Geometry check sheet. Reference: the model listing, model coordinates, mm. Round coordinates to 2 decimals unless told otherwise and drop trailing zeros. Order: outer loops, then holes, each group sorted by start corner. A loop starts at its lowest first (then second) coordinate and runs counter-clockwise, first axis right, second up. Notation, with made-up numbers: (10.5, 20) -> (35.5, 20) arc R30 ccw to (35.5, 54) -> close; hole circle Ø5 at (76.5, 41). An arc over 180 degrees is marked (long way). Use a Markdown table: item, result. Add a question column.
Item 1: Sectioned sample at D-D, the plane x = 47. Record the cut outline in (y, z).
Item 2: Gauge pin test, flat ends, axial feed: pin 1 Ø0.5 at (x, z) = (19, 1) entering from +Y; pin 2 Ø1.5 at (x, z) = (33, 1) entering from -Y. Record the tip position at first contact, or that the pin passes through.
Item 3: Sectioned sample at A-A, the plane x = -30. Record the cut outline in (y, z), and give its area (3 significant figures).
Item 4: Material ranges on probe 1 along X at (y, z) = (4.5, 1.9); probe 2 along X at (y, z) = (-2.5, 2.4); probe 3 along Y at (x, z) = (-30, 1.95), recorded low to high. Write a range as [from, to].
Item 5: Sectioned sample at C-C, the plane x = -11. Record the cut outline in (y, z), and give its area (3 significant figures).
Item 6: Sectioned sample at B-B, the plane z = 1.15. State how many separate pieces and enclosed holes the cut face has, and give its area (3 significant figures).
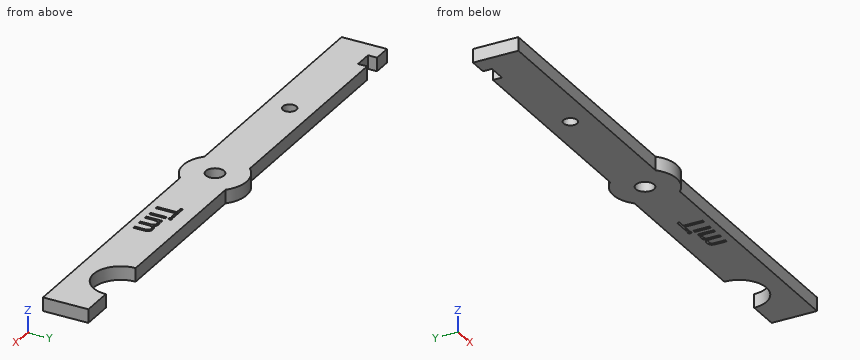
from build123d import *

# Parameters (mm, degrees)
F0_R     = 1.5
F0_R_2   = 2
F0_W     = 0.5472596904
F0_H     = 3.6114921765
F1_DEPTH = 3


with BuildPart() as f1:
    # F0 (on Top) → F1 (new body)
    with BuildSketch(Plane.XY):
        with BuildLine():
            Line((4.8989794856, -5), (-4.8989794856, -5))
            ThreePointArc((-4.8989794856, -5), (0, -7), (4.8989794856, -5))
        make_face()
        with BuildLine():
            ThreePointArc((4.8989794856, 5), (0, 7), (-4.8989794856, 5))
            Line((-4.8989794856, 5), (4.8989794856, 5))
        make_face()
        with BuildLine():
            Line((-60, 5), (-60, -5))
            Line((-60, -5), (-4.8989794856, -5))
            ThreePointArc((-4.8989794856, -5), (-7, 0), (-4.8989794856, 5))
            Line((-4.8989794856, 5), (-52, 5))
            Line((-52, 5), (-52, 3))
            Line((-52, 3), (-56, 3))
            Line((-56, 3), (-56, 5))
            Line((-56, 5), (-60, 5))
        make_face()
        with Locations((-30, 0)):
            Circle(F0_R, mode=Mode.SUBTRACT)
        with BuildLine():
            ThreePointArc((-4.8989794856, 5), (-7, 0), (-4.8989794856, -5))
            Line((-4.8989794856, -5), (4.8989794856, -5))
            ThreePointArc((4.8989794856, -5), (6.4534043883, -2.7117470016), (7, 0))
            ThreePointArc((7, 0), (6.4534043883, 2.7117470016), (4.8989794856, 5))
            Line((4.8989794856, 5), (-4.8989794856, 5))
        make_face()
        Circle(F0_R_2, mode=Mode.SUBTRACT)
        with BuildLine():
            ThreePointArc((7, 0), (6.4534043883, -2.7117470016), (4.8989794856, -5))
            Line((4.8989794856, -5), (60, -5))
            Line((60, -5), (60, 5))
            Line((60, 5), (53, 5))
            ThreePointArc((53, 5), (47, -1), (41, 5))
            Line((41, 5), (4.8989794856, 5))
            ThreePointArc((4.8989794856, 5), (6.4534043883, 2.7117470016), (7, 0))
        make_face()
        with Locations((20.3390103817, -1.4335251428)):
            Rectangle(F0_W, F0_H, mode=Mode.SUBTRACT)
        with BuildLine():
            Line((26.9224706456, -3.239271231), (26.3762654055, -3.239271231))
            Line((26.3762654055, -3.239271231), (26.3762654055, -0.8899560283))
            add(Edge.make_bspline(
                [(26.3762654055, -0.8899560283), (26.3762654055, -0.4576314174), (26.1917366082, -0.2419963371)],
                knots=[0, 0, 0, 1, 1, 1], degree=2))
            add(Edge.make_bspline(
                [(26.1917366082, -0.2419963371), (26.0072078108, -0.0263612568), (25.618115661, -0.0263612568)],
                knots=[0, 0, 0, 1, 1, 1], degree=2))
            add(Edge.make_bspline(
                [(25.618115661, -0.0263612568), (25.1077617301, -0.0263612568), (24.8636564925, -0.319498432)],
                knots=[0, 0, 0, 1, 1, 1], degree=2))
            add(Edge.make_bspline(
                [(24.8636564925, -0.319498432), (24.6195512548, -0.6126356072), (24.6195512548, -1.2221078635)],
                knots=[0, 0, 0, 1, 1, 1], degree=2))
            Line((24.6195512548, -1.2221078635), (24.6195512548, -3.239271231))
            Line((24.6195512548, -3.239271231), (24.0722915645, -3.239271231))
            Line((24.0722915645, -3.239271231), (24.0722915645, -0.8899560283))
            add(Edge.make_bspline(
                [(24.0722915645, -0.8899560283), (24.0722915645, -0.4576314174), (23.8877627671, -0.2419963371)],
                knots=[0, 0, 0, 1, 1, 1], degree=2))
            add(Edge.make_bspline(
                [(23.8877627671, -0.2419963371), (23.7032339698, -0.0263612568), (23.3109784692, -0.0263612568)],
                knots=[0, 0, 0, 1, 1, 1], degree=2))
            add(Edge.make_bspline(
                [(23.3109784692, -0.0263612568), (22.7974611874, -0.0263612568), (22.5586282011, -0.3342607358)],
                knots=[0, 0, 0, 1, 1, 1], degree=2))
            add(Edge.make_bspline(
                [(22.5586282011, -0.3342607358), (22.3197952149, -0.6421602147), (22.3197952149, -1.3444240949)],
                knots=[0, 0, 0, 1, 1, 1], degree=2))
            Line((22.3197952149, -1.3444240949), (22.3197952149, -3.239271231))
            Line((22.3197952149, -3.239271231), (21.7725355245, -3.239271231))
            Line((21.7725355245, -3.239271231), (21.7725355245, 0.3722209455))
            Line((21.7725355245, 0.3722209455), (22.2175135386, 0.3722209455))
            Line((22.2175135386, 0.3722209455), (22.3060873614, -0.1223162314))
            Line((22.3060873614, -0.1223162314), (22.3324486181, -0.1223162314))
            add(Edge.make_bspline(
                [(22.3324486181, -0.1223162314), (22.4874528079, 0.1412963362), (22.7695182552, 0.2899738244)],
                knots=[0, 0, 0, 1, 1, 1], degree=2))
            add(Edge.make_bspline(
                [(22.7695182552, 0.2899738244), (23.0515837026, 0.4386513125), (23.4006067421, 0.4386513125)],
                knots=[0, 0, 0, 1, 1, 1], degree=2))
            add(Edge.make_bspline(
                [(23.4006067421, 0.4386513125), (24.2473303094, 0.4386513125), (24.5077795262, -0.1750387449)],
                knots=[0, 0, 0, 1, 1, 1], degree=2))
            Line((24.5077795262, -0.1750387449), (24.5341407829, -0.1750387449))
            add(Edge.make_bspline(
                [(24.5341407829, -0.1750387449), (24.6954716743, 0.1086083779), (25.0017894779, 0.2736298452)],
                knots=[0, 0, 0, 1, 1, 1], degree=2))
            add(Edge.make_bspline(
                [(25.0017894779, 0.2736298452), (25.3081072815, 0.4386513125), (25.7003627821, 0.4386513125)],
                knots=[0, 0, 0, 1, 1, 1], degree=2))
            add(Edge.make_bspline(
                [(25.7003627821, 0.4386513125), (26.3129983893, 0.4386513125), (26.6177345175, 0.1238979068)],
                knots=[0, 0, 0, 1, 1, 1], degree=2))
            add(Edge.make_bspline(
                [(26.6177345175, 0.1238979068), (26.9224706456, -0.190855499), (26.9224706456, -0.8836293267)],
                knots=[0, 0, 0, 1, 1, 1], degree=2))
            Line((26.9224706456, -0.8836293267), (26.9224706456, -3.239271231))
        make_face(mode=Mode.SUBTRACT)
        Polygon((17.8963763301, 1.0808115273), (17.8963763301, -3.239271231), (17.3364632365, -3.239271231), (17.3364632365, 1.0808115273), (15.810673695, 1.0808115273), (15.810673695, 1.5785120549), (19.4221658715, 1.5785120549), (19.4221658715, 1.0808115273), align=None, mode=Mode.SUBTRACT)
        with BuildLine():
            add(Edge.make_bspline(
                [(20.1112491233, 1.0755392759), (20.0189847246, 1.1662219992), (20.0189847246, 1.3507507965)],
                knots=[0, 0, 0, 1, 1, 1], degree=2))
            add(Edge.make_bspline(
                [(20.0189847246, 1.3507507965), (20.0189847246, 1.5384429447), (20.1112491233, 1.6259623171)],
                knots=[0, 0, 0, 1, 1, 1], degree=2))
            add(Edge.make_bspline(
                [(20.1112491233, 1.6259623171), (20.203513522, 1.7134816896), (20.3427009577, 1.7134816896)],
                knots=[0, 0, 0, 1, 1, 1], degree=2))
            add(Edge.make_bspline(
                [(20.3427009577, 1.7134816896), (20.4745072415, 1.7134816896), (20.569934991, 1.6243806417)],
                knots=[0, 0, 0, 1, 1, 1], degree=2))
            add(Edge.make_bspline(
                [(20.569934991, 1.6243806417), (20.6653627404, 1.5352795939), (20.6653627404, 1.3507507965)],
                knots=[0, 0, 0, 1, 1, 1], degree=2))
            add(Edge.make_bspline(
                [(20.6653627404, 1.3507507965), (20.6653627404, 1.1662219992), (20.569934991, 1.0755392759)],
                knots=[0, 0, 0, 1, 1, 1], degree=2))
            add(Edge.make_bspline(
                [(20.569934991, 1.0755392759), (20.4745072415, 0.9848565527), (20.3427009577, 0.9848565527)],
                knots=[0, 0, 0, 1, 1, 1], degree=2))
            add(Edge.make_bspline(
                [(20.3427009577, 0.9848565527), (20.203513522, 0.9848565527), (20.1112491233, 1.0755392759)],
                knots=[0, 0, 0, 1, 1, 1], degree=2))
        make_face(mode=Mode.SUBTRACT)
    extrude(amount=F1_DEPTH)


solid = f1.part
Found:
| question | item | result |
|---|---|---|
| 1 | outline | (-5, 0) -> (-1, 0) -> (-1, 3) -> (-5, 3) -> close |
| 2 | pin 1 | stops at y = 5 |
| 2 | pin 2 | stops at y = -5 |
| 3 | outline | (-5, 0) -> (-1.5, 0) -> (-1.5, 3) -> (-5, 3) -> close; (1.5, 0) -> (5, 0) -> (5, 3) -> (1.5, 3) -> close |
| 3 | area | 21.0 mm2 |
| 4 | probe 1 | x = [-60, -56], [-52, 41.02], [52.98, 60] |
| 4 | probe 2 | x = [-60, 17.34], [17.9, 20.07], [20.61, 21.77], [22.32, 24.07], [24.62, 26.38], [26.92, 60] |
| 4 | probe 3 | y = [-5, -1.5], [1.5, 5] |
| 5 | outline | (-5, 0) -> (5, 0) -> (5, 3) -> (-5, 3) -> close |
| 5 | area | 30.0 mm2 |
| 6 | separate pieces | 1 |
| 6 | enclosed holes | 6 |
| 6 | area | 1,130 mm2 |
